The figure shows three views and two pictorial views of one solid part (mm, origin at its lowest corner). Answer the questions. A direction names the side the tool comes from. Coordinates: 2 decimals unless noted, no trailing zeros. Write each loop counter-clockwise with the first axis right and the second up, starting at its lowest first coordinate (ties: lowest second). Pieces come first, ordered by that corner, then holes. Notation, with made-up numbers: M -5,85.25 L 51,85.25 A18 ccw 51,106.25 Z; hole C 88.5,7.5 d7. An arc over 180 degrees is marked long. Use CSV: the item, a comma, the result in double quotes.
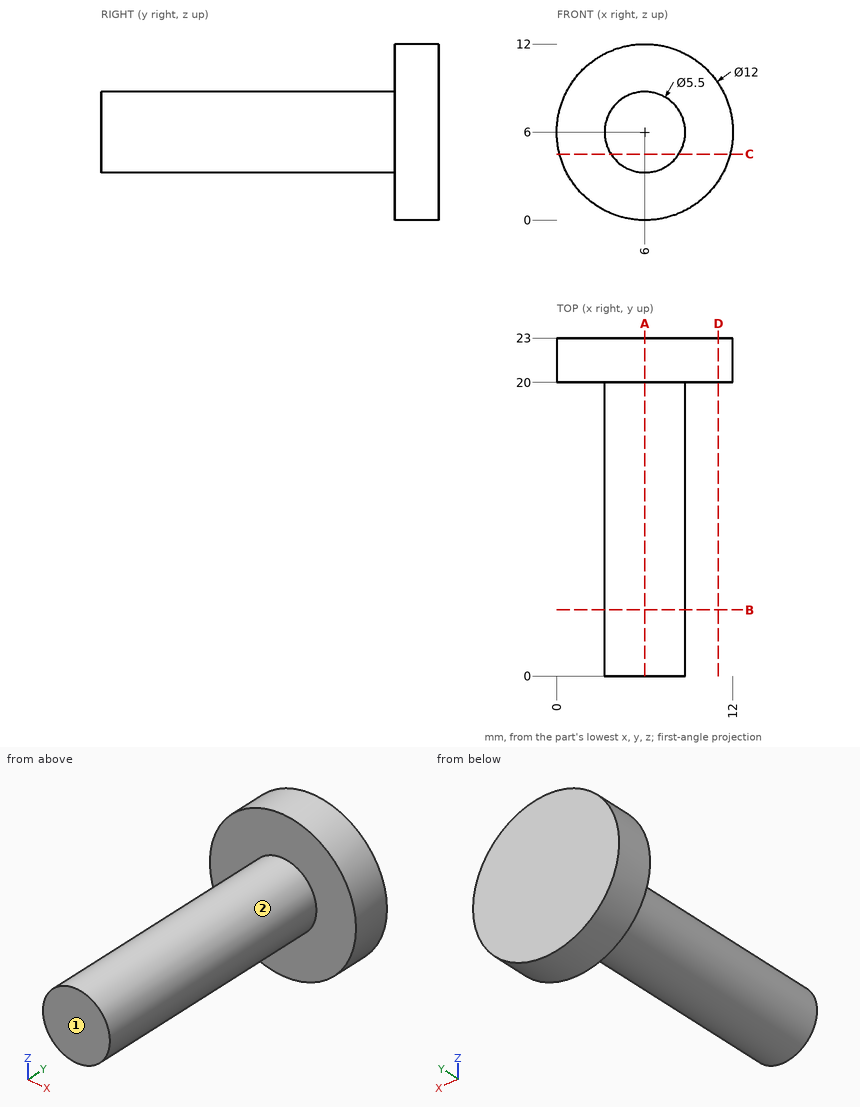
Item 1: Given pin 1 (2 mm diameter, centred on x = 10, y = 19.5, fed in from -Z); pin 2 (1 mm diameter, centred on y = 3, z = 2, fed in from +X); pin 3 (4 mm diameter, centred on x = 8, z = 11, fed in from -Y); pin 4 (6 mm diameter, centred on x = 3, z = 4.5, fed in from -Y), each flat-ended and moving along its own axis, determine where each tip first touches the part or whether it passes through.
Answer:
pin 1,"stops at z = 0.88"
pin 2,"passes through"
pin 3,"stops at y = 20"
pin 4,"stops at y = 0"
Item 2: The part is cut by section D-D (x = 11). Write down the section's boundary in (y, z).
Answer:
outline,"M 20,2.68 L 23,2.68 L 23,9.32 L 20,9.32 Z"
Item 3: The part is cut by section C-C (z = 4.5). Write down the section's boundary in (x, y), then the cut area to 3 significant figures.
Answer:
outline,"M 0.19,20 L 3.7,20 L 3.7,0 L 8.3,0 L 8.3,20 L 11.81,20 L 11.81,23 L 0.19,23 Z"
area,"127 mm2"
Item 4: Consider probe 1 along Y at (x, z) = (2, 2.75); probe 2 along Z at (x, y) = (6.5, 6.25). Determine where each line is inside the solid, lowest interval first.
Answer:
probe 1,"y = 20 to 23"
probe 2,"z = 3.3 to 8.7"
Item 5: The part is cut by section A-A (x = 6). Write down the section's boundary in (y, z).
Answer:
outline,"M 0,3.25 L 20,3.25 L 20,0 L 23,0 L 23,12 L 20,12 L 20,8.75 L 0,8.75 Z"
Item 6: The part is cut by section B-B (y = 4.5). Write down the section's boundary in (x, z), then the cut area to 3 significant figures.
Answer:
outline,"C 6,6 d5.5"
area,"23.8 mm2"
Item 7: A tool of negligible diameter and unlimited length cuts with its end or side. For the marked faces 1 and 2, from which of +Z, -Z, +X, -X, +Y, -Y can it reach the whole face along a straight path? Write none if from no direction.
Answer:
face 1,"+Z, -Z, +X, -X, -Y"
face 2,"-Y"
